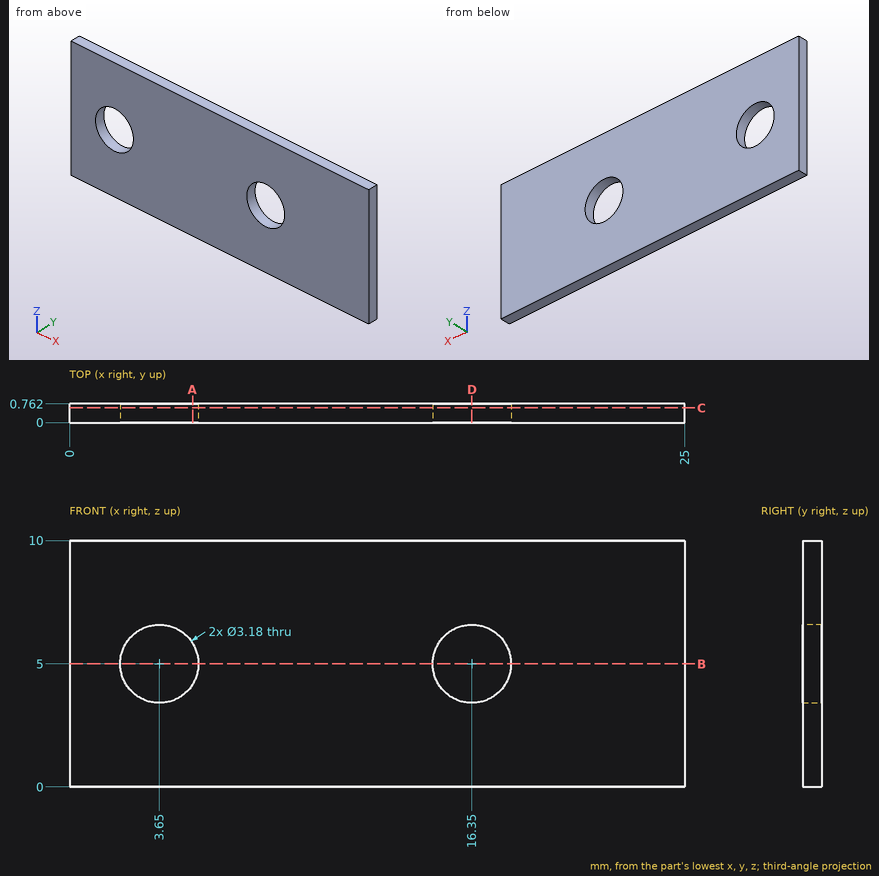
Print and shaded views of the part. All mm, measured from the part's lowest x, y and z. Round coordinates to 2 decimals unless told otherwise and drop trailing zeros. Write each loop counter-clockwise with the first axis right and the second up, starting at its lowest first coordinate (ties: lowest second). Pieces come first, ordered by that corner, then holes. Notation, with made-up numbers: (75, -17.75) - (111, -17.75) arc R37 ccw to (111, 21.25) - close; hole circle Ø5 at (-26.75, 57.25). An arc over 180 degrees is marked (long way). One line per item, written item: value.
(1) Cut at C-C, the plane y = 0.6. Give the cut face in (x, z).
Values follow:
outline: (0, 0) - (25, 0) - (25, 10) - (0, 10) - close; hole circle Ø3.18 at (3.65, 5); hole circle Ø3.18 at (16.35, 5)
(2) Cut at A-A, the plane x = 5. Give the cut face in (y, z), plus the area to 3 significant figures.
Values follow:
outline: (0, 0) - (0.76, 0) - (0.76, 4.16) - (0, 4.16) - close; (0, 5.84) - (0.76, 5.84) - (0.76, 10) - (0, 10) - close
area: 6.34 mm²
(3) Wall check: probe 1 along X at (y, z) = (0.45, 5); probe 2 along X at (y, z) = (0.6, 4.25); probe 3 along Z at (x, y) = (16.35, 0.5). Give the ranges that are in metal, low to high.
Values follow:
probe 1: x = 0 to 2.06, 5.24 to 14.76, 17.94 to 25
probe 2: x = 0 to 2.25, 5.05 to 14.95, 17.75 to 25
probe 3: z = 0 to 3.41, 6.59 to 10
(4) Cut at D-D, the plane x = 16.35. Give the cut face in (y, z), plus the area to 3 significant figures.
Values follow:
outline: (0, 0) - (0.76, 0) - (0.76, 3.41) - (0, 3.41) - close; (0, 6.59) - (0.76, 6.59) - (0.76, 10) - (0, 10) - close
area: 5.20 mm²
(5) Cut at B-B, the plane z = 5. Give the cut face in (x, y), plus the area to 3 significant figures.
Values follow:
outline: (0, 0) - (2.06, 0) - (2.06, 0.76) - (0, 0.76) - close; (5.24, 0) - (14.76, 0) - (14.76, 0.76) - (5.24, 0.76) - close; (17.94, 0) - (25, 0) - (25, 0.76) - (17.94, 0.76) - close
area: 14.2 mm²
